from build123d import *

# Parameters (mm, degrees)
SKETCH1_R            = 60
BOSS_EXTRUDE1_DEPTH  = 5
CUT_EXTRUDE1_DEPTH   = 5
BOSS_EXTRUDE2_DEPTH  = 23
SKETCH4_R            = 3.25
CUT_EXTRUDE2_DEPTH   = 15
BOSS_EXTRUDE3_START  = -5
BOSS_EXTRUDE3_DEPTH  = 5
SKETCH6_W            = 30
SKETCH6_H            = 30
BOSS_EXTRUDE4_DEPTH  = 80
SKETCH10_R           = 14
BOSS_EXTRUDE6_DEPTH  = 3
SKETCH7_W            = 18
SKETCH7_H            = 28
BOSS_EXTRUDE9_DEPTH  = 28
SKETCH15_W           = 14
SKETCH15_H           = 26
CUT_EXTRUDE3_DEPTH   = 26
SKETCH16_W           = 14
SKETCH16_H           = 10
CUT_EXTRUDE4_DEPTH   = 2
SKETCH12_W           = 30
SKETCH12_H           = 100
BOSS_EXTRUDE11_DEPTH = 6
SKETCH17_R           = 3.5
CUT_EXTRUDE5_DEPTH   = 1.5


with BuildPart() as part:
    # Sketch1 → Boss-Extrude1 (new body)
    with BuildSketch(Plane(origin=(0, 0, 0), x_dir=(1, 0, 0), z_dir=(0, 1, 0))):
        with Locations(Location((0, 0, 0), (0, 0, 270))):
            Circle(SKETCH1_R)
    extrude(amount=BOSS_EXTRUDE1_DEPTH)

    # Sketch2 → Cut-Extrude1 (cut)
    with BuildSketch(Plane(origin=(0, 5, 0), x_dir=(1, 0, 0), z_dir=(0, 1, 0))):
        with BuildLine():
            ThreePointArc((-43.005482325, 30.112762908), (-52.5, 0), (-43.005482325, -30.112762908))
            ThreePointArc((-43.005482325, -30.112762908), (-29.078197519, -32.568518988), (-26.622441439, -18.641234181))
            ThreePointArc((-26.622441439, -18.641234181), (-32.5, 0), (-26.622441439, 18.641234181))
            ThreePointArc((-26.622441439, 18.641234181), (-29.078197519, 32.568518988), (-43.005482325, 30.112762908))
        make_face()
        with BuildLine():
            ThreePointArc((43.005482325, 30.112762908), (29.078197519, 32.568518988), (26.622441439, 18.641234181))
            ThreePointArc((26.622441439, 18.641234181), (32.5, 0), (26.622441439, -18.641234181))
            ThreePointArc((26.622441439, -18.641234181), (29.078197519, -32.568518988), (43.005482325, -30.112762908))
            ThreePointArc((43.005482325, -30.112762908), (52.5, 0), (43.005482325, 30.112762908))
        make_face()
    extrude(amount=-CUT_EXTRUDE1_DEPTH, mode=Mode.SUBTRACT)

    # Sketch3 → Boss-Extrude2 (add)
    with BuildSketch(Plane(origin=(0, 5, 0), x_dir=(1, 0, 0), z_dir=(0, 1, 0))):
        with BuildLine():
            Line((10, 56.623758265), (10, 59.160797831))
            ThreePointArc((10, 59.160797831), (0, 60), (-10, 59.160797831))
            Line((-10, 59.160797831), (-10, 56.623758265))
            Line((-10, 56.623758265), (10, 56.623758265))
        make_face()
    extrude(amount=BOSS_EXTRUDE2_DEPTH)

    # Sketch4 → Cut-Extrude2 (cut)
    with BuildSketch(Plane(origin=(0, 5, 0), x_dir=(1, 0, 0), z_dir=(0, 1, 0))):
        with Locations(Location((0, 0, 0), (0, 0, 270))):
            Circle(SKETCH4_R)
    extrude(amount=-CUT_EXTRUDE2_DEPTH, mode=Mode.SUBTRACT)

    # Sketch5 → Boss-Extrude3 (add)
    with BuildSketch(Plane(origin=(0, 5, 0), x_dir=(1, 0, 0), z_dir=(0, 1, 0)).offset(BOSS_EXTRUDE3_START)):
        with BuildLine():
            Line((-58.094750193, 15), (-158.094750193, 15))
            Line((-158.094750193, 15), (-158.094750193, -15))
            Line((-158.094750193, -15), (-58.094750193, -15))
            ThreePointArc((-58.094750193, -15), (-60, 0), (-58.094750193, 15))
        make_face()
    boss_extrude3 = extrude(amount=BOSS_EXTRUDE3_DEPTH)

    # Mirror1: Boss-Extrude3 across plane
    add(boss_extrude3.mirror(Plane(origin=(0, 0, 0), x_dir=(0, 0, 1), z_dir=(1, 0, 0))))

    # Sketch6 → Boss-Extrude4 (add)
    with BuildSketch(Plane.XZ):
        with Locations((-143.094750193, 0)):
            Rectangle(SKETCH6_W, SKETCH6_H)
    boss_extrude4 = extrude(amount=BOSS_EXTRUDE4_DEPTH)

    # Mirror2: Boss-Extrude4 across plane
    add(boss_extrude4.mirror(Plane(origin=(0, 0, 0), x_dir=(0, 0, 1), z_dir=(1, 0, 0))))

    # Sketch10 → Boss-Extrude6 (add)
    with BuildSketch(Plane(origin=(0, 28, 0), x_dir=(1, 0, 0), z_dir=(0, 1, 0))):
        with BuildLine():
            Line((-10, 59.160797831), (-10, 52.168042812))
            ThreePointArc((-10, 52.168042812), (0, 20.973758265), (10, 52.168042812))
            Line((10, 52.168042812), (10, 59.160797831))
            Line((10, 59.160797831), (0, 60))
            Line((0, 60), (-10, 59.160797831))
        make_face()
        with Locations(Location((0, 38.173758265, 0), (0, 0, 270))):
            Circle(SKETCH10_R, mode=Mode.SUBTRACT)
    extrude(amount=BOSS_EXTRUDE6_DEPTH)

    # Sketch7 → Boss-Extrude9 (add)
    with BuildSketch(Plane.XZ):
        with Locations((0, -5.5)):
            Rectangle(SKETCH7_W, SKETCH7_H)
    extrude(amount=BOSS_EXTRUDE9_DEPTH)

    # Sketch15 → Cut-Extrude3 (cut)
    with BuildSketch(Plane.XY.offset(8.5)):
        with Locations((0, -13)):
            Rectangle(SKETCH15_W, SKETCH15_H)
    extrude(amount=-CUT_EXTRUDE3_DEPTH, mode=Mode.SUBTRACT)

    # Sketch16 → Cut-Extrude4 (cut)
    with BuildSketch(Plane.XY.offset(-17.5)):
        with Locations((0, -5)):
            Rectangle(SKETCH16_W, SKETCH16_H)
    extrude(amount=-CUT_EXTRUDE4_DEPTH, mode=Mode.SUBTRACT)

    # Sketch12 → Boss-Extrude11 (add)
    with BuildSketch(Plane.XZ.offset(80)):
        Polygon((128.094750193, 115), (128.094750193, 15), (158.094750193, 15), (158.516628994, 15), (158.516628994, 115), align=None)
        with Locations((143.094750193, -65)):
            Rectangle(SKETCH12_W, SKETCH12_H)
        with Locations((-143.094750193, 65)):
            Rectangle(SKETCH12_W, SKETCH12_H)
        with Locations((-143.094750193, -65)):
            Rectangle(SKETCH12_W, SKETCH12_H)
    extrude(amount=-BOSS_EXTRUDE11_DEPTH)

    # Sketch17 → Cut-Extrude5 (cut)
    with BuildSketch(Plane(origin=(0, 0, -60), x_dir=(-1, 0, 0), z_dir=(0, 0, -1))):
        with Locations((0, 15)):
            Circle(SKETCH17_R)
    extrude(amount=-CUT_EXTRUDE5_DEPTH, mode=Mode.SUBTRACT)


solid = part.part
Model file for the job. Use its own axes, mm. A direction names the side the tool comes from. Give positions to 0.01 mm unless a question says otherwise; leave off trailing zeros. Order: outer loops, then holes, each group sorted by start corner. A loop starts at its lowest first (then second) coordinate and runs counter-clockwise, first axis right, second up. Notation, with made-up numbers: (43.25, 6) - (65.25, 6) arc R20 ccw to (65.25, 11) - close; hole circle Ø9 at (70.25, 2). An arc over 180 degrees is marked (long way). Return JSON: item names as keys, results as strings.
1) Probe line 1 (X direction, y = 15, z = -58.9); line 2 (X direction, y = -72.5, z = -13); line 3 (Y direction, x = 0, z = -59.15). List the from-to ranges inside material, lowest first. Write a range as from..to.
Geometry says:
{"line 1": "-10..-3.5, 3.5..10", "line 2": "-158.09..-128.09, 128.09..158.09", "line 3": "0..11.5, 18.5..31"}
2) Cut at A-A, the plane y = -50. Give the cut face in (x, z), plus the area to 3 significant figures.
Geometry says:
{"outline": "(-158.09, -15) - (-128.09, -15) - (-128.09, 15) - (-158.09, 15) - close; (128.09, -15) - (158.09, -15) - (158.09, 15) - (128.09, 15) - close", "area": "1,800 mm²"}
3) Cut at B-B, the plane y = -18.5. Give the cut face in (x, z).
Geometry says:
{"outline": "(-158.09, -15) - (-128.09, -15) - (-128.09, 15) - (-158.09, 15) - close; (-9, -19.5) - (9, -19.5) - (9, 8.5) - (7, 8.5) - (7, -17.5) - (-7, -17.5) - (-7, 8.5) - (-9, 8.5) - close; (128.09, -15) - (158.09, -15) - (158.09, 15) - (128.09, 15) - close"}
4) Pull direction Z, two halves, no side cores. Call faces 4 (the cylindrical face through (-0.607, 29.479, -20.984)), 5 (the cylindrical face through (28.9, 2.54, 32.44)), 6 (the flat face through (0, -18, -17.5)): pulls with the +Z half, pulls with the -Z half, needs draft (parallel to the pull), parting line crosses it, or undercut.
Geometry says:
{"face 4": "parting line crosses it", "face 5": "undercut", "face 6": "pulls with the +Z half"}
5) 3-axis set-ups, long thin cutter, end or side, ignore diameter. For faces 1 (the flat face through (0, -26, -4)), 2 (the cylindrical face through (0.62, 29.48, -52.16)), 3 (the flat face through (-131, -25, 15)): which of +Z, -Z, +X, -X, +Y, -Y reach the whole face in a straight line?
Geometry says:
{"face 1": "+Z", "face 2": "+Y", "face 3": "+Z, -X, +Y"}
6) Flat gauge pins, fed straight in: P1, Ø4, axis at x = 0.5, z = 1.5, coming from the +Y side; P2, Ø8.5, axis at y = -11, z = -7, coming from the +X side; P3, Ø3, axis at x = -106.5, y = 7, coming from the +Z side; P4, Ø14.5, axis at x = 4.5, y = -9.5, coming from the +Z side. Where does each tip first touch, or does it go through?
Geometry says:
{"P1": "y = 5", "P2": "x = 158.09", "P3": "through", "P4": "z = 8.5"}
7) Cut at D-D, the plane x = 70.5. Give the cut face in (y, z).
Geometry says:
{"outline": "(0, -15) - (5, -15) - (5, 15) - (0, 15) - close"}
8) Cut at C-C, the plane z = 23.5. Give the cut face in (x, y), plus the area to 3 significant figures.
Geometry says:
{"outline": "(-158.09, -80) - (-128.09, -80) - (-128.09, -74) - (-158.09, -74) - close; (-55.21, 0) - (-46.95, 0) - (-46.95, 5) - (-55.21, 5) - close; (-24.85, 0) - (24.85, 0) - (24.85, 5) - (-24.85, 5) - close; (46.95, 0) - (55.21, 0) - (55.21, 5) - (46.95, 5) - close; (128.09, -80) - (158.52, -80) - (158.52, -74) - (128.09, -74) - close", "area": "694 mm²"}
